Verification items for this drawing (mm, ordinates from the low corner). A direction names the side the tool comes from. Give positions to 0.01 mm unless a question says otherwise; leave off trailing zeros. Write each loop counter-clockwise with the first axis right and the second up, starting at its lowest first coordinate (ties: lowest second). Pieces come first, ordered by that corner, then holes. Notation, with made-up numbers: (-8.5, 86) -> (14.5, 86) arc R21 ccw to (14.5, 114) -> close; hole circle Ø1 at (-25.75, 0). An arc over 180 degrees is marked (long way). Answer as a JSON object with one key per item and string values.
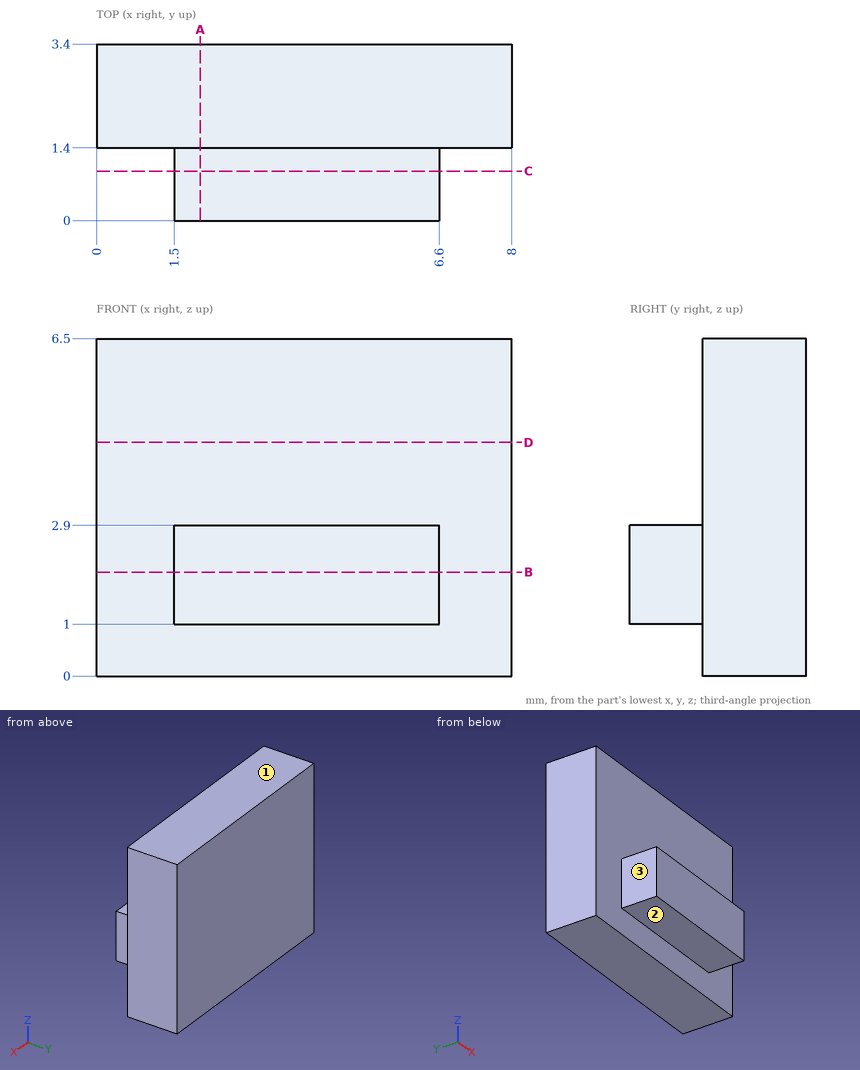
1. Access from +Z, -Z, +X, -X, +Y, -Y to the whole of each face (thin tool, end or side, straight path). Record for the marked faces 1, 2 and 3.
Determined:
{"face 1": "+Z, +X, -X, +Y, -Y", "face 2": "-Z, +X, -X, -Y", "face 3": "+Z, -Z, -X, -Y"}
2. Sectioned sample at A-A, the plane x = 2. Enter the section's corners in (y, z), plus the area to 3 significant figures.
Determined:
{"outline": "(0, 1) -> (1.4, 1) -> (1.4, 0) -> (3.4, 0) -> (3.4, 6.5) -> (1.4, 6.5) -> (1.4, 2.9) -> (0, 2.9) -> close", "area": "15.7 mm^2"}
3. Sectioned sample at D-D, the plane z = 4.5. Enter the section's corners in (x, y).
Determined:
{"outline": "(0, 1.4) -> (8, 1.4) -> (8, 3.4) -> (0, 3.4) -> close"}
4. Sectioned sample at C-C, the plane y = 0.95. Enter the section's corners in (x, z).
Determined:
{"outline": "(1.5, 1) -> (6.6, 1) -> (6.6, 2.9) -> (1.5, 2.9) -> close"}
5. Sectioned sample at B-B, the plane z = 2. Enter the section's corners in (x, y).
Determined:
{"outline": "(0, 1.4) -> (1.5, 1.4) -> (1.5, 0) -> (6.6, 0) -> (6.6, 1.4) -> (8, 1.4) -> (8, 3.4) -> (0, 3.4) -> close"}
6. Scan lines: L1, parallel to Y at x = 1, z = 5.5; L2, parallel to Z at x = 3.5, y = 1.3. Record each from-to range of solid material in increasing order. Write a range as [from, to].
Determined:
{"L1": "[1.4, 3.4]", "L2": "[1, 2.9]"}
7. Go/stop test with flat-tipped pins: P1, Ø1.5, axis at x = 3.5, y = 1, coming from the +Z side; P2, Ø1.5, axis at y = 0.5, z = 1.5, coming from the +X side; P3, Ø3, axis at x = 5.5, z = 4.5, coming from the -Y side; P4, Ø0.7, axis at y = 0.5, z = 2, coming from the -X side. Record where each tip stops, or that it passes through.
Determined:
{"P1": "z = 6.5", "P2": "x = 6.6", "P3": "y = 1.4", "P4": "x = 1.5"}
